CAD build for the part. Positions are in the model's coordinates, mm. A direction names the side the tool comes from. Coordinates: 2 decimals unless noted, no trailing zeros. Write each loop counter-clockwise with the first axis right and the second up, starting at its lowest first coordinate (ties: lowest second). Pieces come first, ordered by that corner, then holes. Notation, with made-up numbers: M 89.25,55.25 L 111.25,55.25 A16 ccw 111.25,70.25 Z; hole C 17.25,61.25 d1. An arc over 180 degrees is marked long. Put each result on its own line as item: value. Start each with the question number.
```python
from build123d import *

# Parameters (mm, degrees)
SALIENTE_EXTRUIR1_DEPTH = 30
VACIADO1_T              = -2
CROQUIS2_W              = 56
CROQUIS2_H              = 5
CROQUIS2_R              = 1.25
SALIENTE_EXTRUIR2_DEPTH = 11


with BuildPart() as part:
    # Croquis1 → Saliente-Extruir1 (new body)
    with BuildSketch(Plane(origin=(0, 0, 0), x_dir=(1, 0, 0), z_dir=(0, 1, 0))):
        with BuildLine():
            Line((-30, 40), (-30, -40))
            ThreePointArc((-30, -40), (-16.865514856, -52.798272284), (0, -60))
            ThreePointArc((0, -60), (16.865514856, -52.798272284), (30, -40))
            Line((30, -40), (30, 40))
            ThreePointArc((30, 40), (15.811388301, 47.434164903), (0, 50))
            ThreePointArc((0, 50), (-15.811388301, 47.434164903), (-30, 40))
        make_face()
    extrude(amount=SALIENTE_EXTRUIR1_DEPTH)

    # Vaciado1
    vaciado1_openings = [part.faces().sort_by_distance(p)[0] for p in [
        (0, 30, 3.068322719),
    ]]
    offset(amount=VACIADO1_T, openings=vaciado1_openings, kind=Kind.INTERSECTION)

    # Croquis2 → Saliente-Extruir2 (add)
    # profile 1 of 2: a face of its own
    with BuildSketch(Plane(origin=(0, 2, 0), x_dir=(1, 0, 0), z_dir=(0, 1, 0))):
        with Locations((0, -31.845)):
            Rectangle(CROQUIS2_W, CROQUIS2_H)
        with Locations(Location((-10.415, -31.845, 0), (0, 0, 270))):
            Circle(CROQUIS2_R, mode=Mode.SUBTRACT)
        with Locations(Location((10.415, -31.845, 0), (0, 0, 270))):
            Circle(CROQUIS2_R, mode=Mode.SUBTRACT)
    # profile 2 of 2: a face of its own
    with BuildSketch(Plane(origin=(0, 2, 0), x_dir=(1, 0, 0), z_dir=(0, 1, 0))):
        with Locations((0, 11.845)):
            Rectangle(CROQUIS2_W, CROQUIS2_H)
        with Locations(Location((-10.415, 11.845, 0), (0, 0, 270))):
            Circle(CROQUIS2_R, mode=Mode.SUBTRACT)
        with Locations(Location((10.415, 11.845, 0), (0, 0, 270))):
            Circle(CROQUIS2_R, mode=Mode.SUBTRACT)
    extrude(amount=SALIENTE_EXTRUIR2_DEPTH)


solid = part.part
```
(1) Two-plate mould, pull along Z, no slides. Class faces 3 (the face through (10, 2, 32)), 4 (the face through (0, 2, -31)), 5 (the face through (16.65, 14.79, 52.94)), 6 (the face through (30, 15, 1)): +Z half, -Z half, draft (parallel to the pull), parting line (faces both ways), or undercut.
(2) Slice it at A-A, the plane y = 16.75. Write the cut outline in (x, z), then the cut area to 3 significant figures.
(3) Slice it at D-D, the plane x = 17. Write the cut outline in (y, z) (3 decimals).
(4) Drill centre lines: line 1 (X direction, y = 16, z = -19.5); line 2 (Z direction, x = -10.5, y = 3.25) (1 decimal); line 3 (Z direction, x = -9, y = 4) (3 decimals). Where is each one in solid material? Low to high. Write a range as [from, to].
(5) Slice it at C-C, the plane y = 4.75. State how many separate pieces and enclosed holes the cut face has, then the cut area to 3 significant figures.
(6) Drop flat-ended pins along their axis: pin 1 (2 mm diameter, centred on x = -11, z = 31.5, fed in from +Y); pin 2 (3 mm diameter, centred on x = 10.5, y = 20.5, fed in from -Z); pin 3 (9 mm diameter, centred on x = -6.5, y = 9.5, fed in from +Z); pin 4 (8 mm diameter, centred on x = 22, z = 28, fed in from -Y). Give the stop position or say it passes through.
(7) Slice it at B-B, the plane z = 11. Write the cut outline in (x, y).
(8) Which spindle directions (+Z, -Z, +X, -X, +Y, -Y) get a long thin tool onto all of the face, cutting with end or side? Do faces 1 (the face through (15.48, 15.804, 51.317)), 2 (the face through (29, 30, 1)). Say none if no direction does.
Result set:
1. face 3: undercut
1. face 4: undercut
1. face 5: +Z half
1. face 6: draft
2. outline: M -30,-40 A50 ccw 30,-40 L 30,40 A50 ccw 0,60 A50 ccw -30,40 Z; hole M -28,-38.99 A48 ccw 28,-38.99 L 28,39.36 A48 ccw 0,57.95 A48 ccw -28,39.36 Z
2. area: 583 mm^2
3. outline: M 0,-47.021 L 30,-47.021 L 30,-44.889 L 2,-44.889 L 2,-14.345 L 13,-14.345 L 13,-9.345 L 2,-9.345 L 2,29.345 L 13,29.345 L 13,34.345 L 2,34.345 L 2,50.276 L 30,50.276 L 30,52.708 L 0,52.708 Z
4. line 1: x = [-30, -28], [28, 30]
4. line 2: z = [-48.9, -46.8], [-14.3, -13.1], [-10.6, -9.3], [29.3, 30.6], [33.1, 34.3], [54.2, 56.4]
4. line 3: z = [-49.183, -47.149], [-14.345, -9.345], [29.345, 34.345], [54.89, 57.078]
5. separate pieces: 1
5. enclosed holes: 7
5. area: 1,120 mm^2
6. pin 1: stops at y = 13
6. pin 2: stops at z = -49.18
6. pin 3: stops at z = 59.51
6. pin 4: stops at y = 0
7. outline: M -30,0 L 30,0 L 30,30 L 28,30 L 28,2 L -28,2 L -28,30 L -30,30 Z
8. face 1: +Y
8. face 2: +Z, -Z, +X, -X, +Y
